Can you work these out from the model? Positions are in its coordinate system, mm. Face numbers are marked on the shaded views. Round coordinates to 2 decimals unless told otherwise and drop trailing zeros. Write each loop counter-clockwise with the first axis right and the second up, starting at its lowest first coordinate (ties: lowest second). Pieces come first, ordered by that corner, then holes. Notation, with made-up numbers: M 82,61 L 105,61 A18 cw 105,75 Z; hole C 32,-8.5 d1. An arc over 180 degrees is marked long. Answer as a JSON object with one key per item and string values. Group by question number.
1) I'm going to push flat-ended pins straight in: pin 1 Ø10 at (x, y) = (2.5, 0) entering from -Z; pin 2 Ø3 at (y, z) = (0, 66.5) entering from +X; pin 3 Ø4 at (y, z) = (-6.5, 23.5) entering from +X; pin 4 Ø1.5 at (x, y) = (6.5, -9.5) entering from -Z. Where does each tip first touch, or does it pass through?
2) Suppose I cut it at B-B, the plane z = 48. Write out the boundary of the cut face in (x, y).
3) If we mould it in two halves opening along Y, with no side actions, what happens to the marked faces 1, 2 and 3? For each: +Y half, -Y half, draft (parallel to the pull), parting line (faces both ways), or undercut.
4) Please list where these lines run through material, in increasing order: L1, parallel to Y at x = 0, z = 18.5; L2, parallel to Y at x = 0, z = 5; L3, parallel to Y at x = 11, z = 15.5. Write a range as [from, to].
5) Suppose I cut it at A-A, the plane z = 25. Write out the boundary of the cut face in (x, y), and give its area (3 significant figures).
from build123d import *

# Parameters (mm, degrees)
F3_DEPTH = 12.7
F4_R     = 5.08


with BuildPart() as f1:
    # F0 (on Front) → F1 (revolve)
    with BuildSketch(Plane.XZ):
        with BuildLine():
            Line((-17.907, 3.175), (-17.907, 0))
            Line((-17.907, 0), (-8.636, 0))
            Line((-8.636, 0), (-8.636, 6.604))
            Line((-8.636, 6.604), (-5.1435, 10.0965))
            Line((-5.1435, 10.0965), (-5.1435, 31.75))
            Line((-5.1435, 31.75), (0, 36.8935))
            Line((0, 36.8935), (0, 79.248))
            Line((0, 79.248), (-5.7601785687, 69.2710780584))
            add(Edge.make_bspline(
                [(-5.7601785687, 69.2710780584), (-10.6664197671, 60.7732190285), (-5.0834936393, 53.2736577196)],
                knots=[0.8570719479, 0.8570719479, 0.8570719479, 2.4112497087, 2.4112497087, 2.4112497087], degree=2, weights=[1, 0.7129578532, 1]))
            ThreePointArc((-5.0834936393, 53.2736577196), (-9.0107667422, 27.5883887463), (-17.907, 3.175))
        make_face()
    revolve(axis=Axis((0, 0, 18.44675), (0, 0, -1)))

    # F2 (on Front) → F3 (cut, symmetric)
    with BuildSketch(Plane.XZ):
        Polygon((7.2810413163, 78.2450328688), (3.175, 79.0126742409), (3.175, 62.9210780584), align=None)
    extrude(amount=F3_DEPTH, both=True, mode=Mode.SUBTRACT)

    # F4
    f4_edges = [f1.edges().sort_by_distance(p)[0] for p in [
        (5.083494, 0, 53.273658),
        (17.907, 0, 3.175),
    ]]
    fillet(f4_edges, radius=F4_R)


solid = f1.part
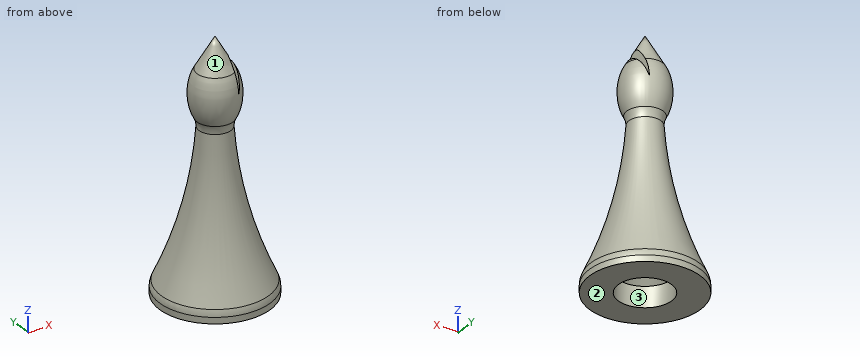
Results:
{
 "1": {"pin 1": "z = 7.74", "pin 2": "x = 7.31", "pin 3": "x = 9.27", "pin 4": "z = 0"},
 "2": {"outline": "C 0,0 d10.94"},
 "3": {"face 1": "parting line", "face 2": "draft", "face 3": "undercut"},
 "4": {"L1": "[-11.69, -5.14], [5.14, 11.69]", "L2": "[-17.05, -8.64], [8.64, 17.05]", "L3": "[-6.41, 6.41]"},
 "5": {"outline": "C 0,0 d19.4; hole C 0,0 d10.29", "area": "213 mm^2"}
}
